Input: part model. Units: mm. Frame: model coordinates. Coordinates: 2 decimals unless noted, no trailing zeros. Loops run counter-clockwise (first coordinate to the right, second up) from the corner with the lowest first, then second, coordinate; pieces in that order, holes last.
(1) Contact query for flat-ended pins moving along their axis: P1, Ø5, axis at y = 104, z = 18.5, coming from the +X side; P2, Ø5, axis at x = -8.5, z = 11, coming from the +Y side; P3, Ø5, axis at y = 101, z = 27.5, coming from the +X side; P4, Ø1, axis at x = -7.5, y = 110, coming from the -Z side. Output: stop coordinate, or through.
(2) Line query: L1, parallel to X at y = 103.25, z = 23.5; L2, parallel to X at y = 105.5, z = 14.5; L3, parallel to Y at x = 1, z = 20.5. Output: solid intervals per line, ascending.
(3) Mould query, pull axis Y, two halves, no side actions, for faces 1 (the face through (0, 105, 0)), 2 (the face through (-0.2, 98.425, 15.653)), 3 (the face through (-10.21, 101.24, 15.65)). Classes: released by +Y, released by -Y, zero draft, split by the parting line, or undercut.
(4) Section A-A, the plane y = 103.25. Return loops of the section in (x, z).
(5) Section D-D, the plane x = 13.5. Return loops of the section in (y, z), then the cut area to 3 significant figures.
(6) Section B-B, the plane z = 6.5. Return loops of the section in (x, y) (3 decimals).
(7) Section C-C, the plane y = 107. Return loops of the section in (x, z).
```python
from build123d import *

# Parameters (mm, degrees)
SKETCH1_R           = 3.175
BOSS_EXTRUDE1_DEPTH = 31.75
FILLET1_R           = 2.54


with BuildPart() as part:
    # Sketch1 → Boss-Extrude1 (new body)
    with BuildSketch(Plane.XY):
        with BuildLine():
            Line((-19.05, 110.768829212), (-16.68220339, 97.000952135))
            ThreePointArc((-16.68220339, 97.000952135), (0, 98.425), (16.68220339, 97.000952135))
            Line((16.68220339, 97.000952135), (19.05, 110.768829212))
            ThreePointArc((19.05, 110.768829212), (0, 112.395), (-19.05, 110.768829212))
        make_face()
        with Locations((9.525, 104.341147205)):
            Circle(SKETCH1_R, mode=Mode.SUBTRACT)
        with Locations((-9.525, 104.341147205)):
            Circle(SKETCH1_R, mode=Mode.SUBTRACT)
    extrude(amount=BOSS_EXTRUDE1_DEPTH)

    # Fillet1
    fillet1_edges = [part.edges().sort_by_distance(p)[0] for p in [
        (19.05, 110.768829212, 15.875),
        (16.68220339, 97.000952135, 15.875),
        (-16.68220339, 97.000952135, 15.875),
        (-19.05, 110.768829212, 15.875),
    ]]
    fillet(fillet1_edges, radius=FILLET1_R)


solid = part.part
```
Report:
1. P1: stops at x = 18.32
1. P2: stops at y = 112.23
1. P3: stops at x = 17.8
1. P4: stops at z = 0
2. L1: x = -17.76 to -12.51, -6.54 to 6.54, 12.51 to 17.76
2. L2: x = -18.14 to -12.48, -6.57 to 6.57, 12.48 to 18.14
2. L3: y = 98.42 to 112.39
3. face 1: zero draft
3. face 2: released by -Y
3. face 3: undercut
4. outline: (-17.76, 0) - (-12.51, 0) - (-12.51, 31.75) - (-17.76, 31.75) - close; (-6.54, 0) - (6.54, 0) - (6.54, 31.75) - (-6.54, 31.75) - close; (12.51, 0) - (17.76, 0) - (17.76, 31.75) - (12.51, 31.75) - close
5. outline: (97.49, 0) - (111.58, 0) - (111.58, 31.75) - (97.49, 31.75) - close
5. area: 447 mm2
6. outline: (-18.615, 108.237) - (-17.107, 99.473) arc R2.54 ccw to (-14.237, 97.39) arc R98.425 cw to (14.237, 97.39) arc R2.54 ccw to (17.107, 99.473) - (18.615, 108.237) arc R2.54 ccw to (16.484, 111.18) arc R112.395 ccw to (-16.484, 111.18) arc R2.54 ccw to start; hole circle Ø6.35 at (-9.525, 104.341); hole circle Ø6.35 at (9.525, 104.341)
7. outline: (-18.4, 0) - (-11.26, 0) - (-11.26, 31.75) - (-18.4, 31.75) - close; (-7.79, 0) - (7.79, 0) - (7.79, 31.75) - (-7.79, 31.75) - close; (11.26, 0) - (18.4, 0) - (18.4, 31.75) - (11.26, 31.75) - close
